from build123d import *

# Parameters (mm, degrees)
SKETCH3_R           = 15
SKETCH3_W           = 80
SKETCH3_H           = 30
BOSS_EXTRUDE2_DEPTH = 20
SKETCH4_W           = 10
SKETCH4_H           = 10
CUT_EXTRUDE1_DEPTH  = 20
CHAMFER1_SIZE       = 40
FILLET1_R           = 2


with BuildPart() as part:
    # Sketch3 → Boss-Extrude2 (new body)
    # profile 1 of 7: a face of its own
    with BuildSketch(Plane.XY):
        Polygon((-80, 75), (-80, 25), (-80, -26.993709631), (-80, -145), (0, -145), (0, 75), align=None)
        with Locations((-30, 0)):
            Circle(SKETCH3_R, mode=Mode.SUBTRACT)
    # profile 2 of 7: a face of its own
    with BuildSketch(Plane.XY):
        Polygon((-80, 75), (-80, 25), (-80, -26.993709631), (-80, -145), (0, -145), (0, 75), align=None)
        with Locations((-30, 0)):
            Circle(SKETCH3_R, mode=Mode.SUBTRACT)
    # profile 3 of 7: a face of its own
    with BuildSketch(Plane.XY):
        Polygon((-80, 75), (-80, 25), (-80, -26.993709631), (-80, -145), (0, -145), (0, 75), align=None)
        with Locations((-30, 0)):
            Circle(SKETCH3_R, mode=Mode.SUBTRACT)
    # profile 4 of 7: a face of its own
    with BuildSketch(Plane.XY):
        with Locations((-40, -160)):
            Rectangle(SKETCH3_W, SKETCH3_H)
    # profile 5 of 7: a face of its own
    with BuildSketch(Plane.XY):
        with Locations((-40, -160)):
            Rectangle(SKETCH3_W, SKETCH3_H)
    # profile 6 of 7: a face of its own
    with BuildSketch(Plane.XY):
        with Locations((-40, -160)):
            Rectangle(SKETCH3_W, SKETCH3_H)
    # profile 7 of 7: a face of its own
    with BuildSketch(Plane.XY):
        Polygon((120, -145), (0, -145), (0, -175), (53.438707699, -175), (120, -175), align=None)
    extrude(amount=BOSS_EXTRUDE2_DEPTH)

    # Sketch4 → Cut-Extrude1 (cut)
    with BuildSketch(Plane.XY.offset(20)):
        with Locations((-65, 60)):
            Rectangle(SKETCH4_W, SKETCH4_H)
        with Locations((-65, 0)):
            Rectangle(SKETCH4_W, SKETCH4_H)
    extrude(amount=-CUT_EXTRUDE1_DEPTH, mode=Mode.SUBTRACT)

    # Chamfer1
    # the kernel refuses this chamfer: 40 mm, written as the material it adds along each edge
    with BuildSketch(Plane(origin=(0, -145, 0), x_dir=(-0.027495876610586535, 0.9996219169112968, 0), z_dir=(0, 0, 1))) as chamfer1_piece_1:
        Polygon((CHAMFER1_SIZE * 0.999621916911, -CHAMFER1_SIZE * 0.0274958766106), (-CHAMFER1_SIZE * 0.0274958766106, -CHAMFER1_SIZE * 0.999621916911), (0, 0), align=None)
    extrude(amount=20)
    # the kernel refuses this chamfer: 40 mm, written as the material it takes off along each edge
    with BuildSketch(Plane(origin=(120, -145, -102.867319519), x_dir=(-0.9996219169112968, 0.027495876610586317, 0), z_dir=(0, 0, 1)), Plane(origin=(0, 75, -102.867319519), x_dir=(-0.9996219169112968, 0.027495876610586317, 0), z_dir=(0, 0, 1))) as chamfer1_2_piece_1:
        Polygon((CHAMFER1_SIZE * 0.999621916911, CHAMFER1_SIZE * 0.0274958766106), (-CHAMFER1_SIZE * 0.0274958766106, CHAMFER1_SIZE * 0.999621916911), (0, 0), align=None)
    extrude(amount=225.734639037, mode=Mode.SUBTRACT)

    # Fillet1
    fillet1_edges = [part.edges().sort_by_distance(p)[0] for p in [
        (-70, 60, 0),
        (-65, 65, 0),
        (-60, 60, 0),
        (-65, 55, 0),
        (-70, 60, 20),
        (-65, 55, 20),
        (-60, 60, 20),
        (-65, 65, 20),
        (-70, 0, 0),
        (-65, 5, 0),
        (-60, 0, 0),
        (-65, -5, 0),
        (-70, 0, 20),
        (-65, -5, 20),
        (-60, 0, 20),
        (-65, 5, 20),
    ]]
    fillet(fillet1_edges, radius=FILLET1_R)


solid = part.part
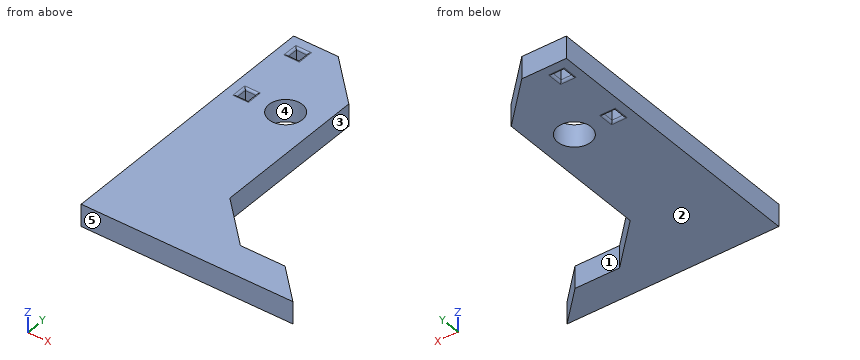
Input: part model. Units: mm. Frame: model coordinates. Face numbers are marked on the shaded views. A direction names the side the tool comes from. Round coordinates to 2 decimals unless told otherwise and drop trailing zeros. Write each loop counter-clockwise with the first axis right and the second up, starting at its lowest first coordinate (ties: lowest second). Pieces come first, ordered by that corner, then holes.
1) Contact query for flat-ended pins moving along their axis: P1, Ø8, axis at y = 1.5, z = 6.5, coming from the +X side; P2, Ø8, axis at x = -6.5, z = 17.5, coming from the +Y side; P3, Ø1.5, axis at y = 37, z = 6.5, coming from the +X side. Output: stop coordinate, or through.
2) Ray query, L1, parallel to Y at x = -30, z = 4.75; L2, parallel to X at y = -107, z = 10; L3, parallel to X at y = 23.5, z = 3.75. Return the intervals inside material, ascending.
3) Cut plane A-A (x = -30). Return the cut outline in (y, z), then the cut area to 3 significant figures.
4) Cut plane C-C (y = 0). Return the cut outline in (x, z).
5) Cut plane D-D (y = -54.5). Return the cut outline in (x, z).
6) Draft query along X for the marked faces 3, 4 and 5. Return one class per face: pulls with the +X half, pulls with the -X half, needs draft (parallel to the pull), parting line crosses it, or undercut.
7) Cut plane B-B (z = 6). Return the cut outline in (x, y).
8) Reachability of the marked faces 1 and 2 from +Z, -Z, +X, -X, +Y, -Y: full face, straight path, thin tool, end or side. Return the list, or none.
Geometry says:
1. P1: stops at x = 0
1. P2: stops at y = 45.5
1. P3: stops at x = -1.25
2. L1: y = -175 to -15, 15 to 65
2. L2: x = -80 to 2
2. L3: x = -80 to 0
3. outline: (-175, 0) - (-15, 0) - (-15, 20) - (-175, 20) - close; (15, 0) - (65, 0) - (65, 20) - (15, 20) - close
3. area: 4,200 mm2
4. outline: (-80, 0) - (-72, 0) arc R2 ccw to (-70, 2) - (-70, 18) arc R2 ccw to (-72, 20) - (-80, 20) - close; (-60, 2) arc R2 ccw to (-58, 0) - (-45, 0) - (-45, 20) - (-58, 20) arc R2 ccw to (-60, 18) - close; (-15, 0) - (0, 0) - (0, 20) - (-15, 20) - close
5. outline: (-80, 0) - (0, 0) - (0, 20) - (-80, 20) - close
6. face 3: pulls with the +X half
6. face 4: undercut
6. face 5: needs draft
7. outline: (-80, -175) - (110, -175) - (80, -145) - (40, -145) - (0, -105) - (0, 35) - (-40, 75) - (-80, 75) - close; hole (-70, -5) - (-60, -5) - (-60, 5) - (-70, 5) - close; hole (-70, 55) - (-60, 55) - (-60, 65) - (-70, 65) - close; hole circle Ø30 at (-30, 0)
8. face 1: +Z, -Z, +X, +Y
8. face 2: -Z, +X, -X, +Y, -Y
